The model under review builds one solid part; all positions refer to its coordinate system, in mm. A direction names the side the tool comes from. Give positions to 0.01 mm unless a question says otherwise; leave off trailing zeros. Order: outer loops, then holes, each group sorted by start corner. A loop starts at its lowest first (then second) coordinate and runs counter-clockwise, first axis right, second up. Notation, with made-up numbers: (-14.75, 36.25) - (-0.75, 36.25) arc R23 ccw to (-0.75, 71.25) - close; hole circle Ø9 at (62.5, -1.5). An arc over 180 degrees is marked (long way). Answer as CSV lines item,"result". Start each with the question number.
from build123d import *

# Parameters (mm, degrees)
SKETCH1_W                = 12
SKETCH1_H                = 10
BOSS_EXTRUDE3_DEPTH      = 3
SKETCH4_W                = 16
SKETCH4_H                = 14
SKETCH4_W_2              = 12
SKETCH4_H_2              = 10
BOSS_EXTRUDE4_DEPTH      = 6
SKETCH5_W                = 16
SKETCH5_H                = 14
BOSS_EXTRUDE5_DEPTH      = 8
M3_CLEARANCE_HOLE1_D     = 3.4
M3_CLEARANCE_HOLE1_DEPTH = 12
M3_CLEARANCE_HOLE1_TIP   = 1.021463052
FILLET1_R                = 4


with BuildPart() as part:
    # Sketch1 → Boss-Extrude3 (new body)
    with BuildSketch(Plane.XY):
        with BuildLine():
            Line((-12.5, 7), (12.5, 7))
            ThreePointArc((12.5, 7), (19.5, 0), (12.5, -7))
            Line((12.5, -7), (-12.5, -7))
            ThreePointArc((-12.5, -7), (-19.5, 0), (-12.5, 7))
        make_face()
        Rectangle(SKETCH1_W, SKETCH1_H, mode=Mode.SUBTRACT)
    extrude(amount=BOSS_EXTRUDE3_DEPTH)

    # Sketch4 → Boss-Extrude4 (add)
    with BuildSketch(Plane.XY.offset(3)):
        Rectangle(SKETCH4_W, SKETCH4_H)
        Rectangle(SKETCH4_W_2, SKETCH4_H_2, mode=Mode.SUBTRACT)
    extrude(amount=BOSS_EXTRUDE4_DEPTH)

    # Sketch5 → Boss-Extrude5 (add)
    with BuildSketch(Plane.XY.offset(9)):
        Rectangle(SKETCH5_W, SKETCH5_H)
        with BuildLine():
            Line((3.31662479, 5), (-3.31662479, 5))
            ThreePointArc((-3.31662479, 5), (-6, 0), (-3.31662479, -5))
            Line((-3.31662479, -5), (3.31662479, -5))
            ThreePointArc((3.31662479, -5), (6, 0), (3.31662479, 5))
        make_face(mode=Mode.SUBTRACT)
    extrude(amount=BOSS_EXTRUDE5_DEPTH)

    # M3 Clearance Hole1
    with Locations(Plane.XY.offset(3)):
        with Locations((-12.5, 0), (12.5, 0)):
            Hole(M3_CLEARANCE_HOLE1_D / 2, depth=M3_CLEARANCE_HOLE1_DEPTH)
            with Locations((0, 0, -(M3_CLEARANCE_HOLE1_DEPTH + M3_CLEARANCE_HOLE1_TIP / 2))):  # 118° drill point
                Cone(0, M3_CLEARANCE_HOLE1_D / 2, M3_CLEARANCE_HOLE1_TIP, mode=Mode.SUBTRACT)

    # Fillet1
    fillet1_edges = [part.edges().sort_by_distance(p)[0] for p in [
        (8, -7, 10),
        (8, 7, 10),
        (-8, 7, 10),
        (-8, -7, 10),
    ]]
    fillet(fillet1_edges, radius=FILLET1_R)


solid = part.part
Item 1: Clearance check with flat-ended pins moving along their axes: pin 1 (5 mm diameter, centred on y = -1, z = 12.5, fed in from +X); pin 2 (3 mm diameter, centred on y = -1.5, z = 11.5, fed in from -X); pin 3 (1.3 mm diameter, centred on x = 4, y = -3, fed in from -Z); pin 4 (2 mm diameter, centred on x = 11.5, y = 4.5, fed in from +Z). State where each tip first meets the part, or that it passes through.
Item 2: Machinability: for faces 1 (the face through (-6.859, -5.797, 10.098)), 2 (the face through (0, -7, 6)), 3 (the face through (5, 4, 9)), 4 (the face through (6.797, -5.859, 10.098)), 5 (the face through (6, 0, 13)), which of the approach directions +Z, -Z, +X, -X, +Y, -Y give a long, thin tool a straight path to every point of the face, cutting with its end or side? Answer none if there is none.
Item 3: Take a section at A-A on x = -5. Write out the cut boundary in (y, z), and give its area (3 significant figures).
Item 4: For line 1 along Y through (x, z) = (-2, 7.5); line 2 along Y through (x, z) = (12.5, 0.95); line 3 along Z through (x, y) = (13, -5), list the stretches that pass through material, from the lowest coordinate up.
Item 5: Take a section at B-B on z = 9.5. Write out the cut boundary in (x, y).
Item 6: Mouldability with a two-part tool opening along Y and no side actions: class faces 6 (the face through (0, -5, 6)), 7 (the face through (-19.5, -0.15, 1.48)), 8 (the face through (-8, 0, 10)) as released by +Y, released by -Y, zero draft, split by the parting line, or undercut.
Item 7: Take a section at C-C on y = -1.25. Write out the cut boundary in (x, z).
Item 8: Take a section at D-D on z = 5.25. Write out the cut boundary in (x, y).
Data:
1,pin 1,"stops at x = 8"
1,pin 2,"stops at x = -8"
1,pin 3,"passes through"
1,pin 4,"stops at z = 3"
2,face 1,"+Z, -X, -Y"
2,face 2,"+Z, -Z, +X, -X, -Y"
2,face 3,"-Z"
2,face 4,"+Z, +X, -Y"
2,face 5,"+Z, -Z"
3,outline,"(-7, 0) - (-5, 0) - (-5, 9) - (-3.32, 9) - (-3.32, 17) - (-6.87, 17) - (-6.87, 3) - (-7, 3) - close; (3.32, 9) - (5, 9) - (5, 0) - (7, 0) - (7, 3) - (6.87, 3) - (6.87, 17) - (3.32, 17) - close"
3,area,"91.4 mm^2"
4,line 1,"y = -7 to -5, 5 to 7"
4,line 2,"y = -7 to -1.7, 1.7 to 7"
4,line 3,"z = 0 to 3"
5,outline,"(-8, -3) arc R4 ccw to (-4, -7) - (4, -7) arc R4 ccw to (8, -3) - (8, 3) arc R4 ccw to (4, 7) - (-4, 7) arc R4 ccw to (-8, 3) - close; hole (-3.32, -5) - (3.32, -5) arc R6 ccw to (3.32, 5) - (-3.32, 5) arc R6 ccw to start"
6,face 6,"undercut"
6,face 7,"split by the parting line"
6,face 8,"zero draft"
7,outline,"(-19.39, 0) - (-13.65, 0) - (-13.65, 3) - (-19.39, 3) - close; (-11.35, 0) - (-6, 0) - (-6, 9) - (-5.87, 9) - (-5.87, 17) - (-8, 17) - (-8, 3) - (-11.35, 3) - close; (5.87, 9) - (6, 9) - (6, 0) - (11.35, 0) - (11.35, 3) - (8, 3) - (8, 17) - (5.87, 17) - close; (13.65, 0) - (19.39, 0) - (19.39, 3) - (13.65, 3) - close"
8,outline,"(-8, -3) arc R4 ccw to (-4, -7) - (4, -7) arc R4 ccw to (8, -3) - (8, 3) arc R4 ccw to (4, 7) - (-4, 7) arc R4 ccw to (-8, 3) - close; hole (-6, -5) - (6, -5) - (6, 5) - (-6, 5) - close"
